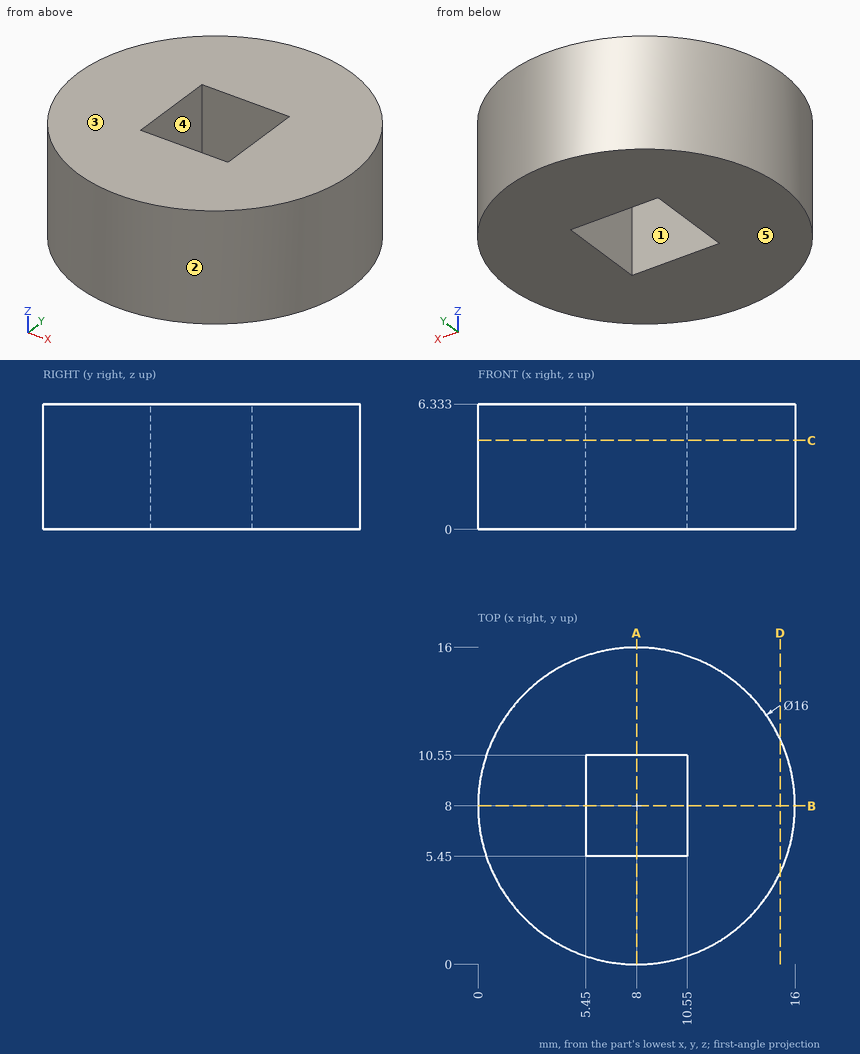
Answer from the drawing. Dimensions are ordinates in mm from the lowest x, y and z of the part. A direction names the side the tool comes from. Round coordinates to 2 decimals unless told otherwise and drop trailing zeros. Loops run counter-clockwise (first coordinate to the right, second up) from the corner with the lowest first, then second, coordinate; pieces in that order, holes last.
1) A cutting plane is placed at C-C on z = 4.5. Determine the outline of the cut face in (x, y).
Outcome:
outline: circle Ø16 at (8, 8); hole (5.45, 5.45) - (10.55, 5.45) - (10.55, 10.55) - (5.45, 10.55) - close
2) A cutting plane is placed at D-D on x = 15.25. Determine the outline of the cut face in (y, z).
Outcome:
outline: (4.62, 0) - (11.38, 0) - (11.38, 6.33) - (4.62, 6.33) - close
3) Given P1, Ø1.5, axis at x = 11, z = 5, coming from the -Y side; P2, Ø2, axis at y = 12.5, z = 5.5, coming from the +X side; P3, Ø1, axis at y = 4.5, z = 3.5, coming from the -X side; P4, Ø4, axis at x = 7, y = 13, coming from the -Z side, each flat-ended and moving along its own axis, determine where each tip first touches the part or whether it passes through.
Outcome:
P1: stops at y = 0.32
P2: stops at x = 15.19
P3: stops at x = 0.58
P4: stops at z = 0
4) A cutting plane is placed at A-A on x = 8. Determine the outline of the cut face in (y, z).
Outcome:
outline: (0, 0) - (5.45, 0) - (5.45, 6.33) - (0, 6.33) - close; (10.55, 0) - (16, 0) - (16, 6.33) - (10.55, 6.33) - close
5) Consider line 1 (Y direction, x = 7.25, z = 5.25); line 2 (Y direction, x = 6.25, z = 3); line 3 (X direction, y = 9.5, z = 5.25). Determine where each line is inside the solid, lowest interval first.
Outcome:
line 1: y = 0.04 to 5.45, 10.55 to 15.96
line 2: y = 0.19 to 5.45, 10.55 to 15.81
line 3: x = 0.14 to 5.45, 10.55 to 15.86
6) For the marked faces 4 and 5, determine the directions among +Z, -Z, +X, -X, +Y, -Y from which every point of the face is accessible in a straight line to the end or side of a thin tool.
Outcome:
face 4: +Z, -Z
face 5: -Z, +X, -X, +Y, -Y
7) For a pull along X with two mould halves and no side action, classify the marked faces 1, 2 and 3 as released by +X, released by -X, zero draft, split by the parting line, or undercut.
Outcome:
face 1: undercut
face 2: split by the parting line
face 3: zero draft
